Source: CAD feature listing. Evaluate the final solid. Frame: model axes, mm. A direction names the side the tool comes from. Round coordinates to 2 decimals unless told otherwise and drop trailing zeros. Loops run counter-clockwise (first coordinate to the right, second up) from the corner with the lowest first, then second, coordinate; pieces in that order, holes last. Notation, with made-up numbers: (11.5, 82.25) - (35.5, 82.25) arc R23 ccw to (35.5, 92.25) - close; hole circle Ø7 at (5.5, 16). An arc over 180 degrees is marked (long way). One line per question, with ' | ' between items. Start each with the question number.
1. Cut plane A-A (x = -3.5). Return loops of the section in (y, z).
2. Pin query (flat end, axial travel): pin 1 (8 mm diameter, centred on x = -7.5, z = -3, fed in from +Y). Return the tip coordinate at first contact, or that it passes through.
3. Mould query, pull axis X, two halves, no side actions, for faces 4 (the flat face through (-8.138, 0.493, -4.908)), 5 (the flat face through (-2.185, 0.493, -7.302)), 6 (the flat face through (8.32, 0.49, -4.59)). Classes: pulls with the +X half, pulls with the -X half, needs draft (parallel to the pull), parting line crosses it, or undercut.
4. Cut plane B-B (y = 4.25). Return loops of the section in (x, z).
5. Cut plane C-C (z = 0). Return loops of the section in (x, y).
6. Ray query, line 1 (X direction, y = 4.35, z = -15); line 2 (Y direction, x = -4.25, z = -7.75); line 3 (X direction, y = 0.65, z = 0). Return the intervals inside material, ascending.
7. Cut plane D-D (x = 0.5). Return loops of the section in (y, z).
8. Access query for faces 1 (the flat face through (0, 6, -15)), 2 (the cylindrical face through (0.6, 3.62, -16.91)), 3 (the cylindrical face through (-7.934, 0.493, 4.553)). Directions: +Z, -Z, +X, -X, +Y, -Y. A direction counts if a zero-diameter tool reaches every point of the face in a straight line with its end or side. Return the directions, or none.
```python
from build123d import *

# Parameters (mm, degrees)
SKETCH1_R           = 4
BOSS_EXTRUDE1_DEPTH = 1
SKETCH3_R           = 2.001662742
BOSS_EXTRUDE2_DEPTH = 6


with BuildPart() as part:
    # Sketch1 → Boss-Extrude1 (new body)
    with BuildSketch(Plane(origin=(0, 0, 0), x_dir=(1, 0, 0), z_dir=(0, 1, 0))):
        with BuildLine():
            Line((-1.733490784, 16.000831371), (-14.723871841, -6.499168629))
            ThreePointArc((-14.723871841, -6.499168629), (-12.472312617, -5.566542262), (-10.988718315, -7.5))
            ThreePointArc((-10.988718315, -7.5), (-11.574991759, -8.915389298), (-12.990381057, -9.501662742))
            Line((-12.990381057, -9.501662742), (12.990381057, -9.501662742))
            ThreePointArc((12.990381057, -9.501662742), (11.256890273, -6.499168629), (14.723871841, -6.499168629))
            Line((14.723871841, -6.499168629), (1.733490784, 16.000831371))
            ThreePointArc((1.733490784, 16.000831371), (1.933457738, 15.518068439), (2.001662742, 15))
            ThreePointArc((2.001662742, 15), (-0.518068439, 13.066542262), (-1.733490784, 16.000831371))
        make_face()
        with BuildLine():
            ThreePointArc((-6.22231578, -5.537682874), (-7.948518941, -4.527622159), (-7.936882283, -2.527656013))
            Line((-7.936882283, -2.527656013), (-6.949410322, -0.840057244))
            ThreePointArc((-6.949410322, -0.840057244), (-6.082439366, -3.464669011), (-4.267076395, -5.549059293))
            Line((-4.267076395, -5.549059293), (-6.22231578, -5.537682874))
        make_face(mode=Mode.SUBTRACT)
        with Locations(Location((0, 0, 0), (0, 0, 270))):
            Circle(SKETCH1_R, mode=Mode.SUBTRACT)
        with BuildLine():
            ThreePointArc((7.906931938, -2.619842099), (7.895295279, -4.619808246), (6.15745546, -5.609713677))
            Line((6.15745546, -5.609713677), (4.202216075, -5.598337258))
            ThreePointArc((4.202216075, -5.598337258), (6.041711062, -3.535212503), (6.939164513, -0.920866911))
            Line((6.939164513, -0.920866911), (7.906931938, -2.619842099))
        make_face(mode=Mode.SUBTRACT)
        with BuildLine():
            ThreePointArc((-1.684616157, 8.157524973), (0.053223662, 9.147430405), (1.779426822, 8.13736969))
            Line((1.779426822, 8.13736969), (2.747194247, 6.438394502))
            ThreePointArc((2.747194247, 6.438394502), (0.040728304, 6.999881514), (-2.672088118, 6.469926204))
            Line((-2.672088118, 6.469926204), (-1.684616157, 8.157524973))
        make_face(mode=Mode.SUBTRACT)
    extrude(amount=BOSS_EXTRUDE1_DEPTH)

    # Sketch3 → Boss-Extrude2 (add)
    with BuildSketch(Plane.XZ):
        with Locations(Location((-12.990381057, 7.5, 0), (0, 0, 270))):
            Circle(SKETCH3_R)
        with Locations(Location((12.990381057, 7.5, 0), (0, 0, 270))):
            Circle(SKETCH3_R)
        with Locations(Location((0, -15, 0), (0, 0, 270))):
            Circle(SKETCH3_R)
    extrude(amount=-BOSS_EXTRUDE2_DEPTH)


solid = part.part
```
Answers follow:
1) outline: (0, -12.94) - (1, -12.94) - (1, -1.94) - (0, -1.94) - close; (0, 1.94) - (1, 1.94) - (1, 9.5) - (0, 9.5) - close
2) pin 1: stops at y = 1
3) face 4: pulls with the -X half | face 5: undercut | face 6: pulls with the +X half
4) outline: circle Ø4 at (-12.99, 7.5); circle Ø4 at (0, -15); circle Ø4 at (12.99, 7.5)
5) outline: (-10.97, 0) - (-4, 0) - (-4, 1) - (-10.97, 1) - close; (4, 0) - (10.97, 0) - (10.97, 1) - (4, 1) - close
6) line 1: x = -2 to 2 | line 2: y = 0 to 1 | line 3: x = -10.97 to -4, 4 to 10.97
7) outline: (0, -16.94) - (6, -16.94) - (6, -13.06) - (1, -13.06) - (1, -9.09) - (0, -9.09) - close; (0, -6.98) - (1, -6.98) - (1, -3.97) - (0, -3.97) - close; (0, 3.97) - (1, 3.97) - (1, 9.5) - (0, 9.5) - close
8) face 1: +Z, -Z, +X, -X, +Y | face 2: +Y | face 3: +Y, -Y
